```python
from build123d import *

# Parameters (mm, degrees)
SKETCH1_R             = 97.5
BOSS_EXTRUDE1_DEPTH   = 28
SKETCH2_R             = 5
CUT_EXTRUDE1_DEPTH    = 141.700035537
SKETCH3_R             = 4.326572982
CUT_EXTRUDE2_DEPTH    = 16.807422
CIRPATTERN1_START     = 11.192577781
CIRPATTERN1_OUTLINE_R = 4.326572982
CIRPATTERN1_DEPTH     = 16.807422219


# Read off the part's stored shape, not the designer's step: CirPattern1
with BuildPart() as part:
    # Sketch1 → Boss-Extrude1 (new body)
    with BuildSketch(Plane(origin=(0, 0, 0), x_dir=(1, 0, 0), z_dir=(0, 1, 0))):
        with Locations(Location((0, 0, 0), (0, 0, 270))):
            Circle(SKETCH1_R)
    extrude(amount=BOSS_EXTRUDE1_DEPTH)

    # Sketch2 → Cut-Extrude1 (cut, through all)
    with BuildSketch(Plane(origin=(0, 0, 0), x_dir=(1, 0, 0), z_dir=(0, 1, 0))):
        with Locations(Location((0, 0, 0), (0, 0, 270))):
            Circle(SKETCH2_R)
    extrude(amount=CUT_EXTRUDE1_DEPTH, mode=Mode.SUBTRACT)

    # Sketch3 → Cut-Extrude2 (cut)
    with BuildSketch(Plane(origin=(0, 28, 0), x_dir=(1, 0, 0), z_dir=(0, 1, 0))):
        with Locations(Location((-41.55757465, 0, 0), (0, 0, 270))):
            Circle(SKETCH3_R)
    extrude(amount=-CUT_EXTRUDE2_DEPTH, mode=Mode.SUBTRACT)

    # CirPattern1 outline → CirPattern1 (cut)
    with BuildSketch(Plane(origin=(0, 0, 0), x_dir=(1, 0, 0), z_dir=(0, 1, 0)).offset(CIRPATTERN1_START)):
        with Locations((-12.841996812, 39.523602172)):
            Circle(CIRPATTERN1_OUTLINE_R)
        with Locations((33.620784137, 24.4269295)):
            Circle(CIRPATTERN1_OUTLINE_R)
        with Locations((33.620784137, -24.4269295)):
            Circle(CIRPATTERN1_OUTLINE_R)
        with Locations((-12.841996812, -39.523602172)):
            Circle(CIRPATTERN1_OUTLINE_R)
    extrude(amount=CIRPATTERN1_DEPTH, mode=Mode.SUBTRACT)


solid = part.part
```
Work out the finished part from the listing and answer in its coordinate system (mm). A direction names the side the tool comes from. Round coordinates to 2 decimals unless told otherwise and drop trailing zeros. Write each loop counter-clockwise with the first axis right and the second up, starting at its lowest first coordinate (ties: lowest second). Pieces come first, ordered by that corner, then holes.
1) A cutting plane is placed at C-C on y = 21. Determine the outline of the cut face in (x, z).
2) A cutting plane is placed at B-B on x = 0. Determine the outline of the cut face in (y, z).
3) A cutting plane is placed at D-D on z = -72. Determine the outline of the cut face in (x, y), and give its area (3 significant figures).
4) Consider probe 1 along X at (y, z) = (18.5, 0); probe 2 along Z at (x, y) = (-10, 16.25); probe 3 along X at (y, z) = (25.5, 3). Determine where each line is inside the solid, lowest interval first.
5) Which of the six approach directions +Z, -Z, +X, -X, +Y, -Y give full straight-line access (tool end or side, diameter ignored) to faces 1 (the face through (-4.88, 13.8, -1.08)), 2 (the face through (34, 11.193, 24))?
6) Determine the mould class of faces 3 (the face through (-86.5, 13.8, 44.99)), 4 (the face through (1, 28, 20)), 5 (the face through (37.748, 19.479, -25.727)) for opening direction X: pulls with the +X half, pulls with the -X half, needs draft (parallel to the pull), parting line crosses it, or undercut.
7) Flat-ended cylindrical pins translate along their axes: P1, Ø7, axis at x = -12.84, z = 39.52, coming from the +Y side; P2, Ø8, axis at x = 0, z = 0, coming from the +Y side; P3, Ø5, axis at y = 9, z = 61.5, coming from the -X side; P4, Ø1, axis at x = 67.5, y = 9.5, coming from the +Z side. Find the tip coordinate at first contact, or state that the pin passes through.
8) A cutting plane is placed at A-A on z = 0. Determine the outline of the cut face in (x, y), and give its area (3 significant figures).
Entries:
1. outline: circle Ø195 at (0, 0); hole circle Ø8.65 at (-41.56, 0); hole circle Ø8.65 at (-12.84, -39.52); hole circle Ø8.65 at (-12.84, 39.52); hole circle Ø10 at (0, 0); hole circle Ø8.65 at (33.62, -24.43); hole circle Ø8.65 at (33.62, 24.43)
2. outline: (0, -97.5) - (28, -97.5) - (28, -5) - (0, -5) - close; (0, 5) - (28, 5) - (28, 97.5) - (0, 97.5) - close
3. outline: (-65.74, 0) - (65.74, 0) - (65.74, 28) - (-65.74, 28) - close
3. area: 3,680 mm2
4. probe 1: x = -97.5 to -45.88, -37.23 to -5, 5 to 97.5
4. probe 2: z = -96.99 to -42.79, -36.26 to 36.26, 42.79 to 96.99
4. probe 3: x = -97.45 to -44.68, -38.44 to -4, 4 to 97.45
5. face 1: +Y, -Y
5. face 2: +Y
6. face 3: parting line crosses it
6. face 4: needs draft
6. face 5: undercut
7. P1: stops at y = 11.19
7. P2: passes through
7. P3: stops at x = -77.62
7. P4: stops at z = 70.83
8. outline: (-97.5, 0) - (-5, 0) - (-5, 28) - (-37.23, 28) - (-37.23, 11.19) - (-45.88, 11.19) - (-45.88, 28) - (-97.5, 28) - close; (5, 0) - (97.5, 0) - (97.5, 28) - (5, 28) - close
8. area: 5,030 mm2
